```python
from build123d import *

# Parameters (mm, degrees)
BOSS_EXTRUDE1_DEPTH             = 5.5
M2_CLEARANCE_HOLE1_D            = 2.4
M2_CLEARANCE_HOLE1_CSINK_D      = 2.45
M2_CLEARANCE_HOLE1_CSINK_ANGLE  = 90
M2X0_4_TAPPED_HOLE1_D           = 1.6
M2X0_4_TAPPED_HOLE1_CSINK_D     = 2.45
M2X0_4_TAPPED_HOLE1_CSINK_ANGLE = 90


with BuildPart() as part:
    # Sketch1 → Boss-Extrude1 (new body)
    with BuildSketch(Plane.XY):
        Polygon((0, 0), (0, 10), (2, 10), (2, 2), (10, 2), (10, 0), align=None)
    extrude(amount=BOSS_EXTRUDE1_DEPTH)

    # M2 Clearance Hole1 (through all)
    with Locations(Plane.ZY):
        with Locations((4, 5)):
            CounterSinkHole(M2_CLEARANCE_HOLE1_D / 2, M2_CLEARANCE_HOLE1_CSINK_D / 2, counter_sink_angle=M2_CLEARANCE_HOLE1_CSINK_ANGLE)

    # M2x0.4 Tapped Hole1 (through all)
    with Locations(Plane(origin=(0, 0, 0), x_dir=(-1, 0, 0), z_dir=(0, -1, 0))):
        with Locations((-5, -4)):
            CounterSinkHole(M2X0_4_TAPPED_HOLE1_D / 2, M2X0_4_TAPPED_HOLE1_CSINK_D / 2, counter_sink_angle=M2X0_4_TAPPED_HOLE1_CSINK_ANGLE)


solid = part.part
```
The listing builds one solid part. Answer for the finished solid, in the listing's coordinates (mm). A direction names the side the tool comes from. Coordinates: 2 decimals unless noted, no trailing zeros. Loops run counter-clockwise (first coordinate to the right, second up) from the corner with the lowest first, then second, coordinate; pieces in that order, holes last. Notation, with made-up numbers: (-30.5, -30) -> (13.5, -30) arc R17 cw to (13.5, 2) -> close; hole circle Ø8 at (-35.75, 7). An arc over 180 degrees is marked (long way). Use one line per item in the form item = value. Start each with the question number.
Item 1: The mould has two halves that part along Y. Classify faces 1 (the face through (1.03, 5.05, 5.2)), 2 (the face through (10, 1, 3)), 3 (the face through (5, 0, 2)): released by +Y, released by -Y, zero draft, split by the parting line, or undercut.
Item 2: Flat-ended cylindrical pins translate along their axes: pin 1 Ø3 at (y, z) = (4.5, 3) entering from +X; pin 2 Ø1.8 at (x, z) = (5, 4) entering from +Y. Find the tip coordinate at first contact, or state that the pin passes through.
Item 3: The part is cut by section B-B on z = 4. Determine the outline of the cut face in (x, y) (3 decimals), then the cut area to 3 significant figures.
Item 4: The part is cut by section C-C on y = 5. Determine the outline of the cut face in (x, z) (3 decimals), then the cut area to 3 significant figures.
Item 5: The part is cut by section A-A on x = 5. Determine the outline of the cut face in (y, z) (3 decimals), then the cut area to 3 significant figures.
Item 6: Consider L1, parallel to Z at x = 0.7, y = 5; L2, parallel to X at y = 1.6, z = 4; L3, parallel to Y at x = 0.8, z = 4. Determine where each line is inside the solid, lowest interval first. Write a range as [from, to].
Item 7: The part is cut by section D-D on y = 1.5. Determine the outline of the cut face in (x, z).
Item 8: A tool of negligible diameter and unlimited length cuts with its end or side. For faces 4 (the face through (2, 6, 3)), 5 (the face through (4.2, 1.2, 4)), from which of +Z, -Z, +X, -X, +Y, -Y can it reach the whole face along a straight path? Write none if from no direction.
Answer key:
q1.face_1 = undercut
q1.face_2 = zero draft
q1.face_3 = released by -Y
q2.pin_1 = 2
q2.pin_2 = 2
q3.outline = (0, 0) -> (3.775, 0) -> (4.2, 0.425) -> (4.2, 2) -> (2, 2) -> (2, 3.8) -> (0.025, 3.8) -> (0, 3.775) -> close; (0, 6.225) -> (0.025, 6.2) -> (2, 6.2) -> (2, 10) -> (0, 10) -> close; (5.8, 0.425) -> (6.225, 0) -> (10, 0) -> (10, 2) -> (5.8, 2) -> close
q3.area = 27.8 mm2
q4.outline = (0, 0) -> (2, 0) -> (2, 2.8) -> (0.025, 2.8) -> (0, 2.775) -> close; (0, 5.225) -> (0.025, 5.2) -> (2, 5.2) -> (2, 5.5) -> (0, 5.5) -> close
q4.area = 6.20 mm2
q5.outline = (0, 0) -> (2, 0) -> (2, 3.2) -> (0.425, 3.2) -> (0, 2.775) -> close; (0, 5.225) -> (0.425, 4.8) -> (2, 4.8) -> (2, 5.5) -> (0, 5.5) -> close
q5.area = 7.62 mm2
q6.L1 = [0, 2.8], [5.2, 5.5]
q6.L2 = [0, 4.2], [5.8, 10]
q6.L3 = [0, 3.8], [6.2, 10]
q7.outline = (0, 0) -> (10, 0) -> (10, 5.5) -> (0, 5.5) -> close; hole circle Ø1.6 at (5, 4)
q8.face_4 = +Z, -Z, +X, +Y
q8.face_5 = +Y, -Y
